Answer from the drawing. Dimensions are ordinates in mm from the lowest x, y and z of the part. Give positions to 0.01 mm unless a question says otherwise; leave off trailing zeros. Order: outer loops, then holes, each group sorted by start corner. A loop starts at its lowest first (then second) coordinate and runs counter-clockwise, first axis right, second up. Notation, with made-up numbers: (59.25, 59.25) - (65.25, 59.25) arc R24 cw to (65.25, 93.25) - close; hole circle Ø3 at (59, 53). An arc over 180 degrees is marked (long way). One line per item, written item: value. Start each with the question number.
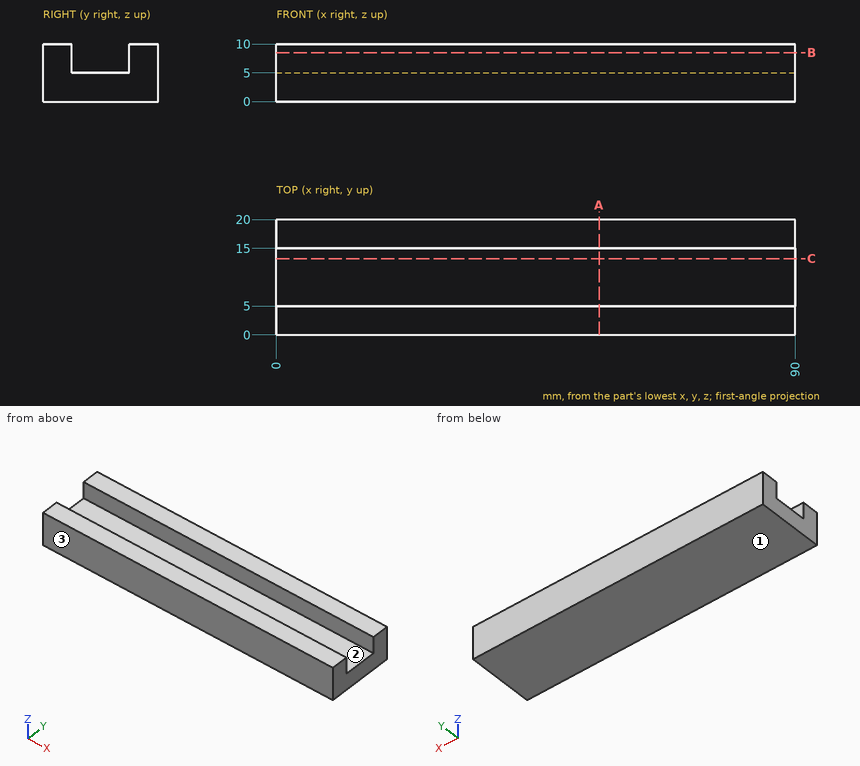
1) Section B-B on z = 8.5 is taken. Write down the section's boundary in (x, y).
2) Section A-A on x = 56 is taken. Write down the section's boundary in (y, z), plus the area to 3 significant figures.
3) The mould has two halves that part along Y. Classify the marked faces 1, 2 and 3: +Y half, -Y half, draft (parallel to the pull), parting line (faces both ways), or undercut.
4) Find the intervals of material crossed by probe 1 along Y at (x, z) = (40, 8.5); probe 2 along Z at (x, y) = (70.5, 12), in increasing order. Write a range as from..to.
5) Section C-C on y = 13.25 is taken. Write down the section's boundary in (x, z), plus the area to 3 significant figures.
6) Each of these flat-tipped pins is pushed along its axis until it touches: pin 1 (1.5 mm diameter, centred on y = 12, z = 6, fed in from +X); pin 2 (5 mm diameter, centred on x = 58.5, y = 11, fed in from +Z). Where does it stop, or does it pass through?
Solved:
1. outline: (0, 0) - (90, 0) - (90, 5) - (0, 5) - close; (0, 15) - (90, 15) - (90, 20) - (0, 20) - close
2. outline: (0, 0) - (20, 0) - (20, 10) - (15, 10) - (15, 5) - (5, 5) - (5, 10) - (0, 10) - close
2. area: 150 mm2
3. face 1: draft
3. face 2: undercut
3. face 3: -Y half
4. probe 1: y = 0..5, 15..20
4. probe 2: z = 0..5
5. outline: (0, 0) - (90, 0) - (90, 5) - (0, 5) - close
5. area: 450 mm2
6. pin 1: passes through
6. pin 2: stops at z = 5
